The figure shows three views and two pictorial views of one solid part (mm, origin at its lowest corner). Answer the questions. A direction names the side the tool comes from. Round coordinates to 2 decimals unless told otherwise and drop trailing zeros. Order: outer loops, then holes, each group sorted by start corner. A loop starts at its lowest first (then second) coordinate and runs counter-clockwise, first axis right, second up.
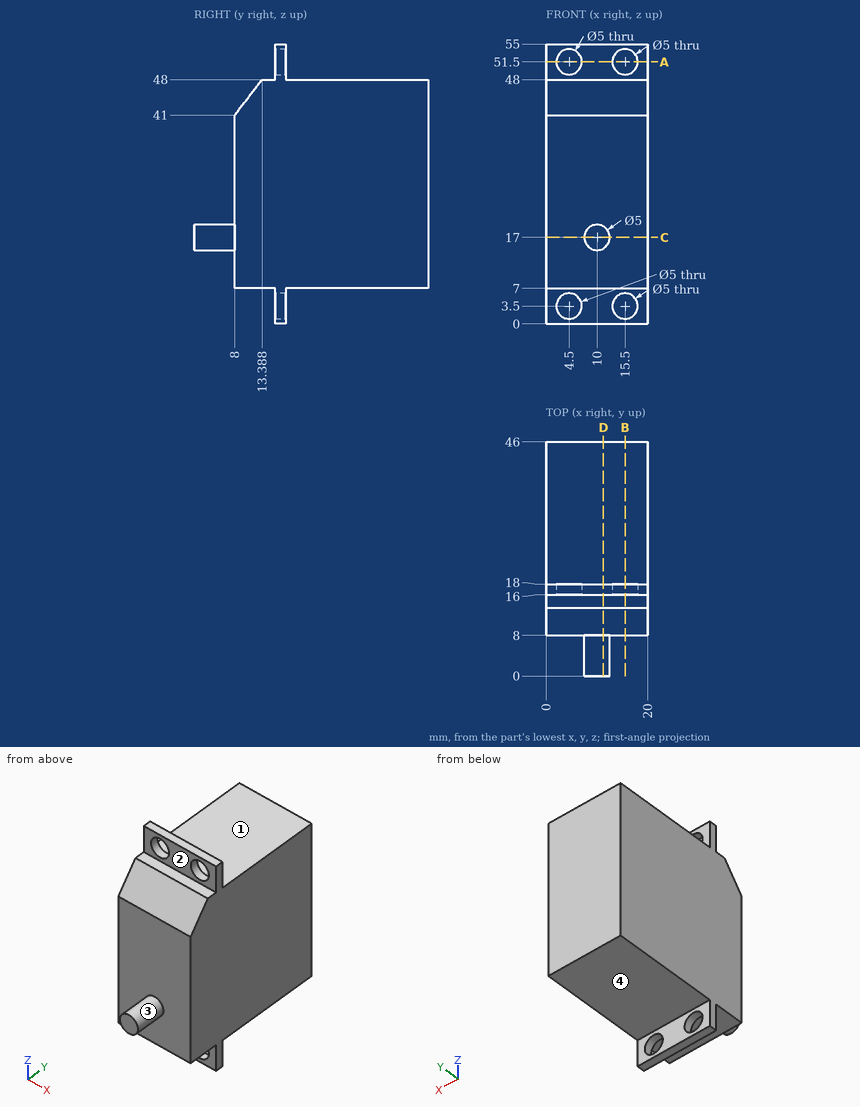
Item 1: Find section C-C (z = 17). Write down the section's boundary in (x, y), plus the area to 3 significant figures.
Item 2: A tool of negligible diameter and unlimited length cuts with its end or side. For the marked faces 1, 2, 3 and 4, from which of +Z, -Z, +X, -X, +Y, -Y can it reach the whole face along a straight path? Write none if from no direction.
Item 3: Given pin 1 (12 mm diameter, centred on x = 4, y = 34, fed in from +Z); pin 2 (8 mm diameter, centred on x = 16.5, y = 30.5, fed in from -Z); pin 3 (5 mm diameter, centred on x = 10.5, z = 41, fed in from -Y), each flat-ended and moving along its own axis, determine where each tip first touches the part or whether it passes through.
Item 4: Find section B-B (x = 15.5). Write down the section's boundary in (y, z).
Item 5: Find section A-A (z = 51.5). Write down the section's boundary in (x, y).
Item 6: Find section D-D (x = 11.25). Write down the section's boundary in (y, z) (1 decimal), plus the area to 3 significant figures.
Item 7: Find the intervals of material crossed by line 1 along X through (y, z) = (17.2, 3.5); line 2 along X through (y, z) = (17, 51); line 3 along Y through (x, z) = (2, 19), in increasing order.
Model answer:
1. outline: (0, 8) - (7.5, 8) - (7.5, 0) - (12.5, 0) - (12.5, 8) - (20, 8) - (20, 46) - (0, 46) - close
1. area: 800 mm2
2. face 1: +Z, +X, -X, +Y
2. face 2: +Z, +X, -X, -Y
2. face 3: -Y
2. face 4: -Z, +X, -X, +Y
3. pin 1: stops at z = 48
3. pin 2: stops at z = 7
3. pin 3: stops at y = 8
4. outline: (8, 7) - (16, 7) - (16, 6) - (18, 6) - (18, 7) - (46, 7) - (46, 48) - (18, 48) - (18, 49) - (16, 49) - (16, 48) - (13.39, 48) - (8, 41) - close; (16, 0) - (18, 0) - (18, 1) - (16, 1) - close; (16, 54) - (18, 54) - (18, 55) - (16, 55) - close
5. outline: (0, 16) - (2, 16) - (2, 18) - (0, 18) - close; (7, 16) - (13, 16) - (13, 18) - (7, 18) - close; (18, 16) - (20, 16) - (20, 18) - (18, 18) - close
6. outline: (0, 14.8) - (8, 14.8) - (8, 7) - (16, 7) - (16, 0) - (18, 0) - (18, 7) - (46, 7) - (46, 48) - (18, 48) - (18, 55) - (16, 55) - (16, 48) - (13.4, 48) - (8, 41) - (8, 19.2) - (0, 19.2) - close
6. area: 1,600 mm2
7. line 1: x = 0 to 2, 7 to 13, 18 to 20
7. line 2: x = 0 to 2.05, 6.95 to 13.05, 17.95 to 20
7. line 3: y = 8 to 46
